For this review, take the finished solid that the model builds, in its own axes (mm). Face numbers are marked on the shaded views. A direction names the side the tool comes from. Give positions to 0.01 mm unless a question says otherwise; leave off trailing zeros. Order: outer loops, then holes, each group sorted by start corner. A loop starts at its lowest first (then second) coordinate and runs counter-clockwise, first axis right, second up. Notation, with made-up numbers: (11, 12.25) - (38, 12.25) arc R23 cw to (38, 26.25) - close; hole circle Ø8 at (89.5, 62). An arc over 180 degrees is marked (long way). One line per item, written item: value.
```python
from build123d import *

# Parameters (mm, degrees)
F0_R     = 5
F1_DEPTH = 4


with BuildPart() as f1:
    # F0 (on Right) → F1 (new body)
    with BuildSketch(Plane.YZ):
        with BuildLine():
            Line((-32.470462, 0), (-11.42762, 0))
            ThreePointArc((-11.42762, 0), (-5.691618, 1.808646), (-2.030496, 6.580344))
            Line((-2.030496, 6.580344), (0, 12.160091))
            Line((0, 12.160091), (1.357265, 15.88982))
            ThreePointArc((1.357265, 15.88982), (1.227999, 16.42686), (0.683047, 16.517132))
            Line((0.683047, 16.517132), (-6.873841, 13.132861))
            Line((-6.873841, 13.132861), (-11.745187, 17))
            Line((-11.745187, 17), (-14.06338, 18.840308))
            ThreePointArc((-14.06338, 18.840308), (-16.302877, 20.073179), (-18.823421, 20.5))
            Line((-18.823421, 20.5), (-34.468871, 20.5))
            ThreePointArc((-34.468871, 20.5), (-39.527112, 22.881214), (-43, 18.5))
            ThreePointArc((-43, 18.5), (-42.106403, 15.808558), (-39.780507, 14.186034))
            ThreePointArc((-39.780507, 14.186034), (-35.001825, 9.308972), (-34.405107, 2.507099))
            ThreePointArc((-34.405107, 2.507099), (-34.053845, 0.778157), (-32.470462, 0))
        make_face()
        with Locations((-18.823421, 12.844194)):
            Circle(F0_R, mode=Mode.SUBTRACT)
    extrude(amount=F1_DEPTH)


solid = f1.part
```
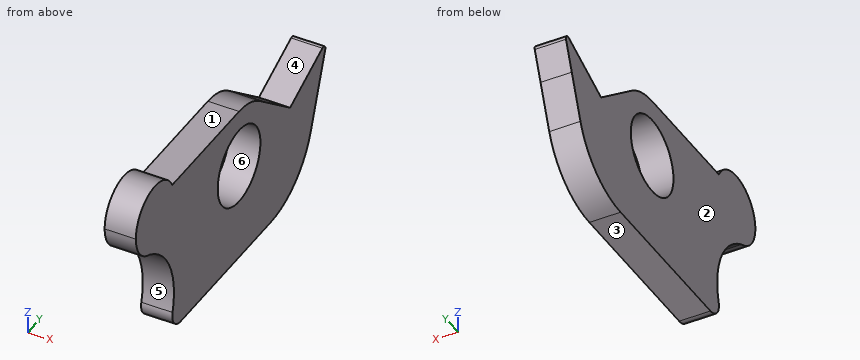
(1) Wall thickness on line 1 (Y direction, x = 2.75, z = 10.5); line 2 (Y direction, x = 3.2, z = 12); line 3 (Z direction, x = 2.9, y = -31): over which ranges is each line inside the solid? List them lowest first. Write a range as from..to.
Answers below:
line 1: y = -35.65..-23.24, -14.41..-0.6
line 2: y = -36.81..-23.75, -13.9..-0.06
line 3: z = 0..20.5
(2) Take a section at A-A (z = 8.5). Write out the cut boundary in (x, y).
Answers below:
outline: (0, -34.67) - (4, -34.67) - (4, -21.3) - (0, -21.3) - close; (0, -16.35) - (4, -16.35) - (4, -1.33) - (0, -1.33) - close
(3) Take a section at D-D (z = 4.5). Write out the cut boundary in (x, y).
Answers below:
outline: (0, -34.09) - (4, -34.09) - (4, -3.08) - (0, -3.08) - close
(4) Take a section at C-C (x = 1.15). Write out the cut boundary in (y, z).
Answers below:
outline: (-43, 18.5) arc R4.5 ccw to (-39.78, 14.19) arc R10.13 cw to (-34.41, 2.51) arc R2 ccw to (-32.47, 0) - (-11.43, 0) arc R10 ccw to (-2.03, 6.58) - (0, 12.16) - (1.36, 15.89) arc R0.5 ccw to (0.68, 16.52) - (-6.87, 13.13) - (-11.75, 17) - (-14.06, 18.84) arc R7.66 ccw to (-18.82, 20.5) - (-34.47, 20.5) arc R4.5 ccw to start; hole circle Ø10 at (-18.82, 12.84)
(5) Draft analysis for pull direction Z (two halves, no side actions). For the marked faces 3, 4, 5 and 6, state which applies: pulls with the +Z half, pulls with the -Z half, needs draft (parallel to the pull), parting line crosses it, or undercut.
Answers below:
face 3: pulls with the -Z half
face 4: pulls with the +Z half
face 5: undercut
face 6: undercut
(6) Machinability: for the marked faces 1 and 2, which of the approach directions +Z, -Z, +X, -X, +Y, -Y give a long, thin tool a straight path to every point of the face, cutting with its end or side? Answer none if there is none.
Answers below:
face 1: +Z, +X, -X, +Y
face 2: +Z, -Z, -X, +Y, -Y
(7) Take a section at B-B (y = -16.5). Write out the cut boundary in (x, z), then the cut area to 3 significant figures.
Answers below:
outline: (0, 0) - (4, 0) - (4, 8.42) - (0, 8.42) - close; (0, 17.27) - (4, 17.27) - (4, 20.14) - (0, 20.14) - close
area: 45.1 mm^2
(8) For P1, Ø2, axis at x = 2.5, y = -26, coming from the +Z side, flat-tipped, find the tip position at first contact; note if it passes through.
Answers below:
P1: stops at z = 20.5
